Here's how the part is built. I have some questions about the finished solid (model axes, mm). Face numbers are marked on the shaded views. A direction names the side the tool comes from. Round coordinates to 2 decimals unless told otherwise and drop trailing zeros. Write each loop counter-clockwise with the first axis right and the second up, starting at its lowest first coordinate (ties: lowest second). Pieces come first, ordered by that corner, then holes. Notation, with made-up numbers: (-39.5, 46.25) -> (-11.5, 46.25) arc R14 ccw to (-11.5, 60.25) -> close; hole circle Ø7 at (24.25, -7). An arc over 180 degrees is marked (long way). Answer as CSV lines item,"result".
from build123d import *

# Parameters (mm, degrees)
F0_W      = 14.75
F0_H      = 14.75
F0_W_2    = 10.25
F0_H_2    = 10.25
F1_DEPTH  = 14.5200116
F2_W      = 14.75
F2_H      = 14.75
F2_W_2    = 10.25
F2_H_2    = 10.25
F3_DEPTH  = 14.5200116
F5_W      = 14.75
F5_H      = 14.5200116
F4_W      = 14.75
F4_H      = 14.5200116
F6_DEPTH  = 17.695037
F7_W      = 14.75
F7_H      = 14.75
F7_W_2    = 10.25
F7_H_2    = 10.25
F8_DEPTH  = 14.5200116
F9_R      = 1.6
F10_DEPTH = 25.4
F11_R     = 1.6
F12_DEPTH = 10
F13_R     = 1.6
F14_DEPTH = 10


with BuildPart() as f1:
    # F0 (on Top) → F1 (new body)
    with BuildSketch(Plane.XY):
        with Locations((5.125, -5.125)):
            Rectangle(F0_W, F0_H)
        with Locations((5.125, -5.125)):
            Rectangle(F0_W_2, F0_H_2, mode=Mode.SUBTRACT)
    extrude(amount=F1_DEPTH)

    # F2 (on face) → F3 (join)
    with BuildSketch(Plane(origin=(0, 0, 0), x_dir=(1, 0, 0), z_dir=(0, 0, -1))):
        with Locations((5.125, 5.125)):
            Rectangle(F2_W, F2_H)
        with Locations((5.125, 5.125)):
            Rectangle(F2_W_2, F2_H_2, mode=Mode.SUBTRACT)
        with Locations((5.125, 5.125)):
            Rectangle(F2_W_2, F2_H_2)
    extrude(amount=F3_DEPTH)

    # F5 (on face) + F4 (on face) → F6 (join)
    with BuildSketch(Plane.XZ.offset(12.5)):
        with Locations((5.125, -7.2600058)):
            Rectangle(F5_W, F5_H)
    with BuildSketch(Plane.XZ.offset(12.5)):
        with Locations((5.125, -7.2600058)):
            Rectangle(F4_W, F4_H)
        Polygon((0, -12.2700116), (0, -2.25), (10.25, -2.25), (10.25, -12.2700116), (10.25, -12.5), (0, -12.5), align=None, mode=Mode.SUBTRACT)
        Polygon((10.25, -2.25), (0, -2.25), (0, -12.2700116), (0, -12.5), (10.25, -12.5), (10.25, -12.2700116), align=None)
    extrude(amount=F6_DEPTH)

    # F7 (on face) → F8 (join)
    with BuildSketch(Plane.XY):
        with Locations((5.125, -22.820037)):
            Rectangle(F7_W, F7_H)
        with Locations((5.125, -22.820037)):
            Rectangle(F7_W_2, F7_H_2, mode=Mode.SUBTRACT)
    extrude(amount=F8_DEPTH)

    # F9 (on face) → F10 (cut)
    with BuildSketch(Plane.YZ.offset(12.5)):
        with Locations((-22.820037, 4.75)):
            Circle(F9_R)
        with Locations((-5.125, 4.75)):
            Circle(F9_R)
    extrude(amount=-F10_DEPTH, mode=Mode.SUBTRACT)

    # F11 (on face) → F12 (cut)
    with BuildSketch(Plane.XZ.offset(30.195037)):
        with Locations((5.125, 4.75)):
            Circle(F11_R)
    extrude(amount=-F12_DEPTH, mode=Mode.SUBTRACT)

    # F13 (on face) → F14 (cut)
    with BuildSketch(Plane(origin=(0, 2.25, 0), x_dir=(-1, 0, 0), z_dir=(0, 1, 0))):
        with Locations((-5.125, 4.75)):
            Circle(F13_R)
    extrude(amount=-F14_DEPTH, mode=Mode.SUBTRACT)


solid = f1.part
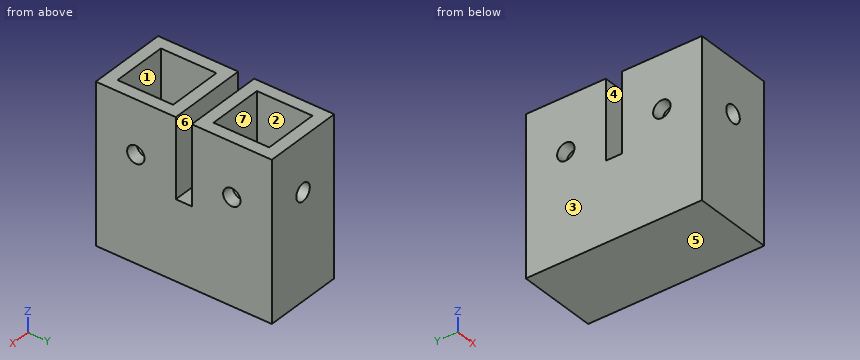
Item 1: Suppose I cut it at A-A, the plane z = 8. List the corners of the cut face in (x, y) for me, then the cut area to 3 significant figures.
Results found:
outline,"(-2.25, -30.2) -> (12.5, -30.2) -> (12.5, -15.45) -> (-2.25, -15.45) -> close; (-2.25, -12.5) -> (12.5, -12.5) -> (12.5, 2.25) -> (-2.25, 2.25) -> close; hole (0, -27.95) -> (10.25, -27.95) -> (10.25, -17.7) -> (0, -17.7) -> close; hole (0, -10.25) -> (10.25, -10.25) -> (10.25, 0) -> (0, 0) -> close"
area,"225 mm²"
Item 2: Suppose I cut it at D-D, the plane x = 2. List the corners of the cut face in (y, z) for me, then the cut area to 3 significant figures.
Results found:
outline,"(-30.2, -14.52) -> (2.25, -14.52) -> (2.25, 14.52) -> (0, 14.52) -> (0, 0) -> (-10.25, 0) -> (-10.25, 14.52) -> (-12.5, 14.52) -> (-12.5, 0) -> (-15.45, 0) -> (-15.45, 14.52) -> (-17.7, 14.52) -> (-17.7, 0) -> (-27.95, 0) -> (-27.95, 14.52) -> (-30.2, 14.52) -> close"
area,"602 mm²"
Item 3: Will this pin go through, and if not, where does the flat tip stop? pin 1 (2.5 mm diameter, centred on y = -5.125, z = 4.75, fed in from -X).
Results found:
pin 1,"passes through"
Item 4: If we mould it in two halves opening along X, with no side actions, what happens to the marked faces 1, 2, 3 and 4? For each: pulls with the +X half, pulls with the -X half, needs draft (parallel to the pull), parting line crosses it, or undercut.
Results found:
face 1,"undercut"
face 2,"undercut"
face 3,"pulls with the -X half"
face 4,"needs draft"
Item 5: For the marked faces 5, 6 and 7, which set-ups out of +Z, -Z, +X, -X, +Y, -Y let a thin tool reach every point of the face, with its end or its side?
Results found:
face 5,"-Z, +X, -X, +Y, -Y"
face 6,"+Z, +X, -X"
face 7,"+Z"
Item 6: I need wall thicknesses on L1, parallel to Y at x = 4.25, z = 10.5; L2, parallel to Z at x = 7.25, y = -3.5; L3, parallel to X at y = -27, z = 7.75. Which ranges of each line are inside material? Lowest first, please.
Results found:
L1,"y = -30.2 to -27.95, -17.7 to -15.45, -12.5 to -10.25, 0 to 2.25"
L2,"z = -14.52 to 0"
L3,"x = -2.25 to 0, 10.25 to 12.5"
Item 7: Suppose I cut it at B-B, the plane y = -20.5. List the corners of the cut face in (x, z) for me.
Results found:
outline,"(-2.25, -14.52) -> (12.5, -14.52) -> (12.5, 14.52) -> (10.25, 14.52) -> (10.25, 0) -> (0, 0) -> (0, 14.52) -> (-2.25, 14.52) -> close"
Item 8: Suppose I cut it at C-C, the plane x = 5.75. List the corners of the cut face in (y, z) for me.
Results found:
outline,"(-30.2, -14.52) -> (2.25, -14.52) -> (2.25, 3.28) -> (0, 3.28) -> (0, 0) -> (-10.25, 0) -> (-10.25, 14.52) -> (-12.5, 14.52) -> (-12.5, 0) -> (-15.45, 0) -> (-15.45, 14.52) -> (-17.7, 14.52) -> (-17.7, 0) -> (-27.95, 0) -> (-27.95, 3.28) -> (-30.2, 3.28) -> close; (-30.2, 6.22) -> (-27.95, 6.22) -> (-27.95, 14.52) -> (-30.2, 14.52) -> close; (0, 6.22) -> (2.25, 6.22) -> (2.25, 14.52) -> (0, 14.52) -> close"
